Geometry: final body of the model. Coordinates: model frame, mm. Coordinates: 2 decimals unless noted, no trailing zeros. Order: outer loops, then holes, each group sorted by start corner. A loop starts at its lowest first (then second) coordinate and runs counter-clockwise, first axis right, second up. Notation, with made-up numbers: (10, -1.5) -> (61, -1.5) arc R25 cw to (61, 11.5) -> close; hole circle Ø4 at (74.5, 78.25). An arc over 180 degrees is marked (long way). Use one line per item in the form item = value.
```python
from build123d import *

# Parameters (mm, degrees)
F0_W     = 40
F0_H     = 40
F0_W_2   = 37
F0_H_2   = 37
F1_DEPTH = 1200
F3_DEPTH = 40


with BuildPart() as f1:
    # F0 (on Front) → F1 (new body, symmetric)
    with BuildSketch(Plane.XZ):
        Rectangle(F0_W, F0_H)
        Rectangle(F0_W_2, F0_H_2, mode=Mode.SUBTRACT)
    extrude(amount=F1_DEPTH, both=True)

    # F2 (on face) → F3 (cut)
    with BuildSketch(Plane.YZ.offset(20)):
        Polygon((1200, -20), (1200, 20), (1160, -20), align=None)
        Polygon((-1160, -20), (-1200, 20), (-1200, -20), align=None)
    extrude(amount=-F3_DEPTH, mode=Mode.SUBTRACT)


solid = f1.part
```
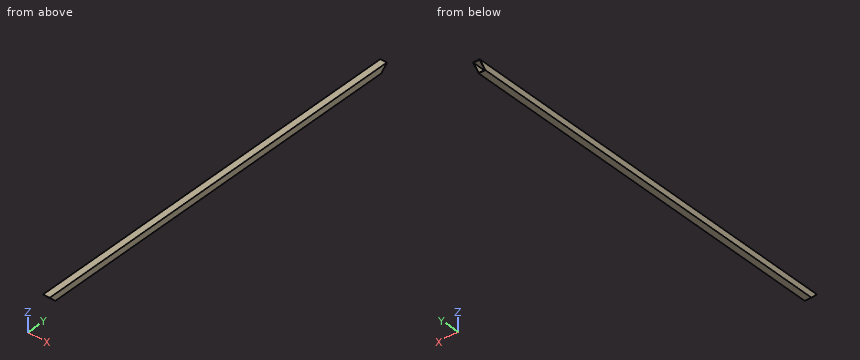
1) Section B-B, the plane y = -801.5. Output: boundary loops of the cut face in (x, z), and give its area (3 significant figures).
Results found:
outline = (-20, -20) -> (20, -20) -> (20, 20) -> (-20, 20) -> close; hole (-18.5, -18.5) -> (18.5, -18.5) -> (18.5, 18.5) -> (-18.5, 18.5) -> close
area = 231 mm2
2) Contact query for a flat-ended pin moving along its axis: P1, Ø5, axis at x = 14.5, z = -12.5, coming from the -Y side. Output: stop coordinate, or through.
Results found:
P1 = through
3) Material intervals for probe 1 along Z at (x, y) = (5.5, 127), sorted ascending. Write a range as from..to.
Results found:
probe_1 = -20..-18.5, 18.5..20
4) Section A-A, the plane z = -2. Output: boundary loops of the cut face in (x, y), and give its area (3 significant figures).
Results found:
outline = (-20, -1178) -> (-18.5, -1178) -> (-18.5, 1178) -> (-20, 1178) -> close; (18.5, -1178) -> (20, -1178) -> (20, 1178) -> (18.5, 1178) -> close
area = 7,070 mm2
5) Section C-C, the plane x = 2.5. Output: boundary loops of the cut face in (y, z), and give its area (3 significant figures).
Results found:
outline = (-1200, 20) -> (-1198.5, 18.5) -> (1198.5, 18.5) -> (1200, 20) -> close; (-1161.5, -18.5) -> (-1160, -20) -> (1160, -20) -> (1161.5, -18.5) -> close
area = 7,080 mm2
